```python
from build123d import *

# Parameters (mm, degrees)
F0_R      = 1.4732
F1_DEPTH  = 3.175
F2_R      = 1.5875
F3_DEPTH  = 3.175
F5_DEPTH  = 2.38125
F6_R      = 2.38125
F7_DEPTH  = 17.4625
F8_R      = 1.4732
F9_DEPTH  = 6.35
F11_R     = 1.4732
F12_DEPTH = 1.5875


with BuildPart() as f1:
    # F0 (on Front) → F1 (new body)
    with BuildSketch(Plane.XZ):
        with BuildLine():
            ThreePointArc((30.9057507299, 33.2053364545), (30.8777447649, 32.9082655755), (30.868397212, 32.6100239545))
            ThreePointArc((30.868397212, 32.6100239545), (30.8777447649, 32.3117823335), (30.9057507299, 32.0147114545))
            ThreePointArc((30.9057507299, 32.0147114545), (35.630897212, 27.8475239545), (40.3560436941, 32.0147114545))
            ThreePointArc((40.3560436941, 32.0147114545), (40.3840496591, 32.3117823335), (40.393397212, 32.6100239545))
            ThreePointArc((40.393397212, 32.6100239545), (40.3840496591, 32.9082655755), (40.3560436941, 33.2053364545))
            ThreePointArc((40.3560436941, 33.2053364545), (35.630897212, 37.3725239545), (30.9057507299, 33.2053364545))
        make_face()
        with BuildLine():
            Line((32.4807995573, 45.7068989545), (30.9057507299, 33.2053364545))
            ThreePointArc((30.9057507299, 33.2053364545), (35.630897212, 37.3725239545), (40.3560436941, 33.2053364545))
            Line((40.3560436941, 33.2053364545), (38.7809948668, 45.7068989545))
            ThreePointArc((38.7809948668, 45.7068989545), (38.7996655101, 45.5088517018), (38.805897212, 45.3100239545))
            ThreePointArc((38.805897212, 45.3100239545), (35.4320694647, 42.1412556564), (32.4807995573, 45.7068989545))
        make_face()
        with BuildLine():
            ThreePointArc((38.7809948668, 45.7068989545), (35.630897212, 48.4850239545), (32.4807995573, 45.7068989545))
            ThreePointArc((32.4807995573, 45.7068989545), (35.4320694647, 42.1412556564), (38.805897212, 45.3100239545))
            ThreePointArc((38.805897212, 45.3100239545), (38.7996655101, 45.5088517018), (38.7809948668, 45.7068989545))
        make_face()
        with Locations((35.630897212, 45.3100239545)):
            Circle(F0_R, mode=Mode.SUBTRACT)
        with Locations((35.630897212, 45.3100239545)):
            Circle(F0_R)
    extrude(amount=F1_DEPTH)

    # F2 (on face) → F3 (join)
    with BuildSketch(Plane(origin=(0, 0, 0), x_dir=(-1, 0, 0), z_dir=(0, 1, 0))):
        with Locations((-35.630897212, 45.3100239545)):
            Circle(F2_R)
    extrude(amount=F3_DEPTH)

    # F4 (on face) → F5 (join)
    with BuildSketch(Plane(origin=(0, 3.175, 0), x_dir=(-1, 0, 0), z_dir=(0, 1, 0))):
        Polygon((-34.5753285935, 42.7710785747), (-32.904321705, 44.9547005036), (-33.9598903235, 47.4936458835), (-36.6864658305, 47.8489693343), (-38.357472719, 45.6653474054), (-37.3019041005, 43.1264020256), align=None)
    extrude(amount=F5_DEPTH)

    # F6 (on face) → F7 (join)
    with BuildSketch(Plane.XZ.offset(3.175)):
        with Locations((35.630897212, 32.6100239545)):
            Circle(F6_R)
    extrude(amount=F7_DEPTH)

    # F8 (on face) → F9 (join)
    with BuildSketch(Plane.XZ.offset(20.6375)):
        with BuildLine():
            ThreePointArc((40.3560436941, 32.0147114545), (40.3840496591, 32.3117823335), (40.393397212, 32.6100239545))
            ThreePointArc((40.393397212, 32.6100239545), (35.332655591, 37.3631764016), (30.9057507299, 32.0147114545))
            ThreePointArc((30.9057507299, 32.0147114545), (35.630897212, 27.8475239545), (40.3560436941, 32.0147114545))
        make_face()
        with BuildLine():
            ThreePointArc((40.3560436941, 32.0147114545), (35.630897212, 27.8475239545), (30.9057507299, 32.0147114545))
            Line((30.9057507299, 32.0147114545), (32.4807995573, 19.5131489545))
            ThreePointArc((32.4807995573, 19.5131489545), (35.4320694647, 23.0787922526), (38.805897212, 19.9100239545))
            ThreePointArc((38.805897212, 19.9100239545), (38.7996655101, 19.7111962072), (38.7809948668, 19.5131489545))
            Line((38.7809948668, 19.5131489545), (40.3560436941, 32.0147114545))
        make_face()
        with BuildLine():
            ThreePointArc((38.805897212, 19.9100239545), (35.4320694647, 23.0787922526), (32.4807995573, 19.5131489545))
            ThreePointArc((32.4807995573, 19.5131489545), (35.630897212, 16.7350239545), (38.7809948668, 19.5131489545))
            ThreePointArc((38.7809948668, 19.5131489545), (38.7996655101, 19.7111962072), (38.805897212, 19.9100239545))
        make_face()
        with Locations((35.630897212, 19.9100239545)):
            Circle(F8_R, mode=Mode.SUBTRACT)
    extrude(amount=F9_DEPTH)

    # F11 (on offset) → F12 (cut, symmetric)
    with BuildSketch(Plane.XZ.offset(23.8125)):
        with BuildLine():
            Line((38.7809948668, 19.5131489545), (39.4310150177, 24.6725239545))
            Line((39.4310150177, 24.6725239545), (31.8307794063, 24.6725239545))
            Line((31.8307794063, 24.6725239545), (32.4807995573, 19.5131489545))
            ThreePointArc((32.4807995573, 19.5131489545), (35.630897212, 16.7350239545), (38.7809948668, 19.5131489545))
        make_face()
        with Locations((35.630897212, 19.9100239545)):
            Circle(F11_R, mode=Mode.SUBTRACT)
    extrude(amount=F12_DEPTH, both=True, mode=Mode.SUBTRACT)


solid = f1.part
```
Can you work these out from the model? Positions are in its coordinate system, mm. A direction names the side the tool comes from. Round coordinates to 2 decimals unless told otherwise and drop trailing zeros. Loops run counter-clockwise (first coordinate to the right, second up) from the corner with the lowest first, then second, coordinate; pieces in that order, holes last. Notation, with made-up numbers: M 73,42 L 97,42 A31 ccw 97,73 Z; hole C 58,-33 d10. An arc over 180 degrees is marked long. Answer in a Markdown table with one row per item.
1. If we section it at C-C, the plane z = 36: Please give me the cut outline in (x, y) (1 decimal).
Established:
| item | result |
|---|---|
| outline | M 31.3,-3.2 L 40,-3.2 L 40,0 L 31.3,0 Z; M 32.3,-27 L 39,-27 L 39,-20.6 L 32.3,-20.6 Z |
2. Thinking about a two-plate mould opening in Z: for faces 1 (the face through (35.3, 4.35, 47.67)), 2 (the face through (36, -20.638, 27)), 3 (the face through (34.55, -21.42, 20.91)), which applies, pulls with the +Z half, pulls with the -Z half, needs draft (parallel to the pull), parting line crosses it, or undercut?
Established:
| item | result |
|---|---|
| face 1 | pulls with the +Z half |
| face 2 | needs draft |
| face 3 | undercut |
3. On a 3-axis mill with a long thin cutter (end or side, diameter ignored), from which of +Z, -Z, +X, -X, +Y, -Y can I reach the whole of each face in a straight line? I mean faces 4 (the face through (36, -25.4, 22)), 5 (the face through (33.75, 4.35, 43.85)), 6 (the face through (37.51, 4.35, 46.77)), 7 (the face through (34.9, 1.6, 43.9)), 8 (the face through (33.425, 4.349, 46.206)). Say none if no direction works.
Established:
| item | result |
|---|---|
| face 4 | -Z, +X, -X |
| face 5 | -Z, -X, +Y |
| face 6 | +Z, +X, +Y |
| face 7 | none |
| face 8 | +Z, -X, +Y |
4. If we section it at A-A, the plane z = 22: Please give me the cut outline in (x, y) (1 decimal), plus the area to 3 significant figures.
Established:
| item | result |
|---|---|
| outline | M 32.2,-27 L 39.1,-27 L 39.1,-25.4 L 32.2,-25.4 Z; M 32.2,-22.2 L 39.1,-22.2 L 39.1,-20.6 L 32.2,-20.6 Z |
| area | 22.0 mm² |
5. Please list where these lines run through material, in increasing order: line 1 (Y direction, x = 34, z = 35.5) (1 decimal); line 2 (Y direction, x = 37, z = 43.5) (3 decimals); line 3 (Y direction, x = 35.25, z = 27). Write a range as from..to.
Established:
| item | result |
|---|---|
| line 1 | -27..-20.6, -3.2..0 |
| line 2 | -3.175..0, 3.175..5.556 |
| line 3 | -26.99..-20.64 |
6. If we section it at D-D, the plane y = -14: Please give me the cut outline in (x, z), plus the area to 3 significant figures.
Established:
| item | result |
|---|---|
| outline | C 35.63,32.61 d4.76 |
| area | 17.8 mm² |
7. I'm going to push flat-ended pins straight in: pin 1 Ø2 at (y, z) = (-16.5, 33.5) entering from -X; pin 2 Ø5 at (x, z) = (36, 40) entering from +Y; pin 3 Ø1.6 at (x, y) = (36.5, -23.5) entering from -Z. Where does each tip first touch, or does it pass through?
Established:
| item | result |
|---|---|
| pin 1 | x = 33.25 |
| pin 2 | y = 0 |
| pin 3 | z = 24.67 |
